Part model, mm, in its own coordinate system. A direction names the side the tool comes from. Give positions to 0.01 mm unless a question says otherwise; leave off trailing zeros. Write each loop counter-clockwise with the first axis right and the second up, starting at its lowest first coordinate (ties: lowest second). Pieces come first, ordered by that corner, then holes. Notation, with made-up numbers: (-2, 66) - (15, 66) arc R24 cw to (15, 86) - close; hole circle Ø7 at (-16, 3). An arc over 180 degrees is marked (long way). Answer as a JSON object with one key per item and string values. Group by question number.
```python
from build123d import *

# Parameters (mm, degrees)
BOSS_EXTRUDE1_DEPTH        = 50
SKETCH2_R                  = 30
CUT_EXTRUDE1_DEPTH         = 30
SKETCH3_R                  = 20
BOSS_EXTRUDE2_DEPTH        = 30
F_20_0MM_DOWEL_HOLE1_D     = 20
F_20_0MM_DOWEL_HOLE1_DEPTH = 30
F_20_0MM_DOWEL_HOLE1_TIP   = 6.00860619
SKETCH6_R                  = 10
CUT_EXTRUDE2_DEPTH         = 109
SKETCH7_R                  = 10
CUT_EXTRUDE3_DEPTH         = 10
BOSS_EXTRUDE3_DEPTH        = 30
SKETCH11_R                 = 5
CUT_EXTRUDE4_DEPTH         = 30
SKETCH13_R                 = 5
CUT_EXTRUDE5_DEPTH         = 20
SKETCH14_W                 = 17
SKETCH14_H                 = 5
BOSS_EXTRUDE4_DEPTH        = 20
SKETCH15_W                 = 91.222515674
SKETCH15_H                 = 40
CUT_EXTRUDE6_DEPTH         = 20
CUT_EXTRUDE7_DEPTH         = 20


with BuildPart() as part:
    # Sketch1 → Boss-Extrude1 (new body)
    with BuildSketch(Plane(origin=(0, 0, 0), x_dir=(1, 0, 0), z_dir=(0, 1, 0))):
        with BuildLine():
            Line((-6.666666667, 39.440531887), (-65, 29.580398915))
            ThreePointArc((-65, 29.580398915), (-74.494747679, 26.265991124), (-82.360679775, 20))
            ThreePointArc((-82.360679775, 20), (-90, 0), (-82.360679775, -20))
            ThreePointArc((-82.360679775, -20), (-74.494747679, -26.265991124), (-65, -29.580398915))
            Line((-65, -29.580398915), (-6.666666667, -39.440531887))
            ThreePointArc((-6.666666667, -39.440531887), (-3.345050411, -39.859887578), (0, -40))
            ThreePointArc((0, -40), (40, 0), (0, 40))
            ThreePointArc((0, 40), (-3.345050411, 39.859887578), (-6.666666667, 39.440531887))
        make_face()
    extrude(amount=BOSS_EXTRUDE1_DEPTH)

    # Sketch2 → Cut-Extrude1 (cut)
    with BuildSketch(Plane.XZ):
        Circle(SKETCH2_R)
    extrude(amount=-CUT_EXTRUDE1_DEPTH, mode=Mode.SUBTRACT)

    # Sketch3 → Boss-Extrude2 (add)
    with BuildSketch(Plane(origin=(0, 50, 0), x_dir=(1, 0, 0), z_dir=(0, 1, 0))):
        Circle(SKETCH3_R)
    extrude(amount=BOSS_EXTRUDE2_DEPTH)

    # Ø20.0mm Dowel Hole1
    with Locations(Plane.ZX.offset(80)):
        with Locations((0, 0)):
            Hole(F_20_0MM_DOWEL_HOLE1_D / 2, depth=F_20_0MM_DOWEL_HOLE1_DEPTH)
            with Locations((0, 0, -(F_20_0MM_DOWEL_HOLE1_DEPTH + F_20_0MM_DOWEL_HOLE1_TIP / 2))):  # 118° drill point
                Cone(0, F_20_0MM_DOWEL_HOLE1_D / 2, F_20_0MM_DOWEL_HOLE1_TIP, mode=Mode.SUBTRACT)

    # Sketch6 → Cut-Extrude2 (cut)
    with BuildSketch(Plane(origin=(0, 50, 0), x_dir=(1, 0, 0), z_dir=(0, 1, 0))):
        with Locations((-60, 0)):
            Circle(SKETCH6_R)
    extrude(amount=-CUT_EXTRUDE2_DEPTH, mode=Mode.SUBTRACT)

    # Sketch7 → Cut-Extrude3 (cut)
    with BuildSketch(Plane(origin=(0, 50, 0), x_dir=(1, 0, 0), z_dir=(0, 1, 0))):
        with BuildLine():
            ThreePointArc((-60, -20), (-40, 0), (-60, 20))
            Line((-60, 20), (-82.360679775, 20))
            ThreePointArc((-82.360679775, 20), (-90, 0), (-82.360679775, -20))
            Line((-82.360679775, -20), (-60, -20))
        make_face()
        with Locations((-60, 0)):
            Circle(SKETCH7_R, mode=Mode.SUBTRACT)
    extrude(amount=-CUT_EXTRUDE3_DEPTH, mode=Mode.SUBTRACT)

    # Sketch10 → Boss-Extrude3 (add)
    with BuildSketch(Plane.XZ):
        with BuildLine():
            Line((20, 60), (0, 40))
            ThreePointArc((0, 40), (28.284271247, 28.284271247), (40, 0))
            Line((40, 0), (60, 20))
            ThreePointArc((60, 20), (60, 60), (20, 60))
        make_face()
    extrude(amount=-BOSS_EXTRUDE3_DEPTH)

    # Sketch11 → Cut-Extrude4 (cut)
    with BuildSketch(Plane(origin=(0, 0, 0), x_dir=(-1, 0, 0), z_dir=(0, -1, 0))):
        with Locations((-40, -40)):
            Circle(SKETCH11_R)
    extrude(amount=-CUT_EXTRUDE4_DEPTH, mode=Mode.SUBTRACT)

    # Sketch13 → Cut-Extrude5 (cut)
    with BuildSketch(Plane(origin=(0, 0, 0), x_dir=(-1, 0, 0), z_dir=(0, -1, 0))):
        with BuildLine():
            ThreePointArc((-68.228756555, -38.228756555), (-60, -60), (-38.228756555, -68.228756555))
            Line((-38.228756555, -68.228756555), (0, -30))
            ThreePointArc((0, -30), (-21.213203436, -21.213203436), (-30, 0))
            Line((-30, 0), (-68.228756555, -38.228756555))
        make_face()
        with Locations((-40, -40)):
            Circle(SKETCH13_R, mode=Mode.SUBTRACT)
    extrude(amount=-CUT_EXTRUDE5_DEPTH, mode=Mode.SUBTRACT)

    # Sketch14 → Boss-Extrude4 (add)
    with BuildSketch(Plane(origin=(0, 50, 0), x_dir=(1, 0, 0), z_dir=(0, 1, 0))):
        with Locations((-28.343134833, 0)):
            Rectangle(SKETCH14_W, SKETCH14_H)
    extrude(amount=BOSS_EXTRUDE4_DEPTH)

    # Sketch15 → Cut-Extrude6 (cut)
    with BuildSketch(Plane.XZ):
        with Locations((-60, 0)):
            Rectangle(SKETCH15_W, SKETCH15_H)
    extrude(amount=-CUT_EXTRUDE6_DEPTH, mode=Mode.SUBTRACT)

    # Sketch16 → Cut-Extrude7 (cut)
    with BuildSketch(Plane.XY.offset(2.5)):
        Polygon((-19.843134833, 70), (-36.843134833, 50), (-36.843134833, 70), align=None)
    extrude(amount=-CUT_EXTRUDE7_DEPTH, mode=Mode.SUBTRACT)


solid = part.part
```
1) Band-saw the part on D-D (x = 24). List the corners of the cut face in (y, z), plus the area to 3 significant figures.
2) Mould opens along Z. For faces 5 (the flat face through (19, 10, 49)), 6 (the flat face through (10, 15, 50)), 7 (the cylindrical face through (60, 21, 60)), 8 (the cylindrical face through (-9.76, 64.79, 2.17)) say: pulls with the +Z half, pulls with the -Z half, needs draft (parallel to the pull), parting line crosses it, or undercut.
3) Drop flat-ended pins along their axis: P1, Ø3, axis at x = -4, y = 71.5, coming from the -Z side; P2, Ø5, axis at y = 58.5, z = -8, coming from the -X side; P3, Ø13, axis at x = 40, z = 40, coming from the -Y side; P4, Ø3, axis at y = 63.5, z = -22, coming from the +X side. Give the stop position or say it passes through.
4) Band-saw the part on A-A (y = 18). List the corners of the cut face in (x, z).
5) Band-saw the part on B-B (y = 27). List the corners of the cut face in (x, z), plus the area to 3 significant figures.
6) Band-saw the part on C-C (z = 43). List the corners of the cut face in (x, y), plus the area to 3 significant figures.
7) Which spindle directions (+Z, -Z, +X, -X, +Y, -Y) get a long thin tool onto all of the face, cutting with end or side? Do faces 1 (the cylindrical face through (13.843, 18.123, -26.615)), 2 (the flat face through (-53, 10, -20)), 3 (the flat face through (-25, 55, -2.5)), 4 (the cylindrical face through (-40, 45, 0)). Say none if no direction does.
8) Probe line 1 (Z direction, x = 0, y = 68); line 2 (Z direction, x = -12.5, y = 10.5); line 3 (Y direction, x = -54.5, z = -29). List the from-to ranges inside material, lowest first.
Verdict:
{
 "1": {"outline": "(0, -32) - (50, -32) - (50, 32) - (30, 32) - (30, 63.32) - (0, 63.32) - (0, 54) - (20, 54) - (20, 18) - (30, 18) - (30, -18) - (0, -18) - close", "area": "2,340 mm2"},
 "2": {"face 5": "undercut", "face 6": "pulls with the +Z half", "face 7": "parting line crosses it", "face 8": "undercut"},
 "3": {"P1": "z = -19.84", "P2": "x = -19.23", "P3": "y = 20", "P4": "through"},
 "4": {"outline": "(-82.36, -20) arc R30 ccw to (-65, -29.58) - (-6.67, -39.44) arc R40 ccw to (40, 0) - (60, 20) arc R28.28 ccw to (68.23, 38.23) - (30, 0) arc R30 cw to (-22.36, -20) - close; (-82.36, 20) - (-22.36, 20) arc R30 cw to (0, 30) - (38.23, 68.23) arc R28.28 ccw to (20, 60) - (0, 40) arc R40 ccw to (-6.67, 39.44) - (-65, 29.58) arc R30 ccw to start"},
 "5": {"outline": "(-65, -29.58) - (-6.67, -39.44) arc R40 ccw to (40, 0) - (60, 20) arc R28.28 ccw to (20, 60) - (0, 40) arc R40 ccw to (-6.67, 39.44) - (-65, 29.58) arc R30 ccw to start; hole circle Ø20 at (-60, 0); hole circle Ø60 at (0, 0); hole circle Ø10 at (40, 40)", "area": "7,370 mm2"},
 "6": {"outline": "(3, 0) - (13, 0) - (13, 20) - (36, 20) - (36, 30) - (3, 30) - close; (44, 20) - (68.12, 20) - (68.12, 30) - (44, 30) - close", "area": "771 mm2"},
 "7": {"face 1": "-Y", "face 2": "-X, -Y", "face 3": "-Z, -X, +Y", "face 4": "-X, +Y"},
 "8": {"line 1": "-20 to -10, 10 to 20", "line 2": "-38.45 to -27.27, 27.27 to 38.45", "line 3": "0 to 50"}
}
